Can you work these out from the drawing? Everything is in mm from the part's minimum corner. A direction names the side the tool comes from. Round coordinates to 2 decimals unless told otherwise and drop trailing zeros. Loops run counter-clockwise (first coordinate to the right, second up) from the corner with the lowest first, then second, coordinate; pieces in that order, holes last. Notation, with made-up numbers: M 65.25,-18.5 L 95.25,-18.5 A18 ccw 95.25,9.5 Z; hole C 77.25,12.25 d7. An arc over 180 degrees is marked long. One line per question, with ' | ' between items. Start each with the question number.
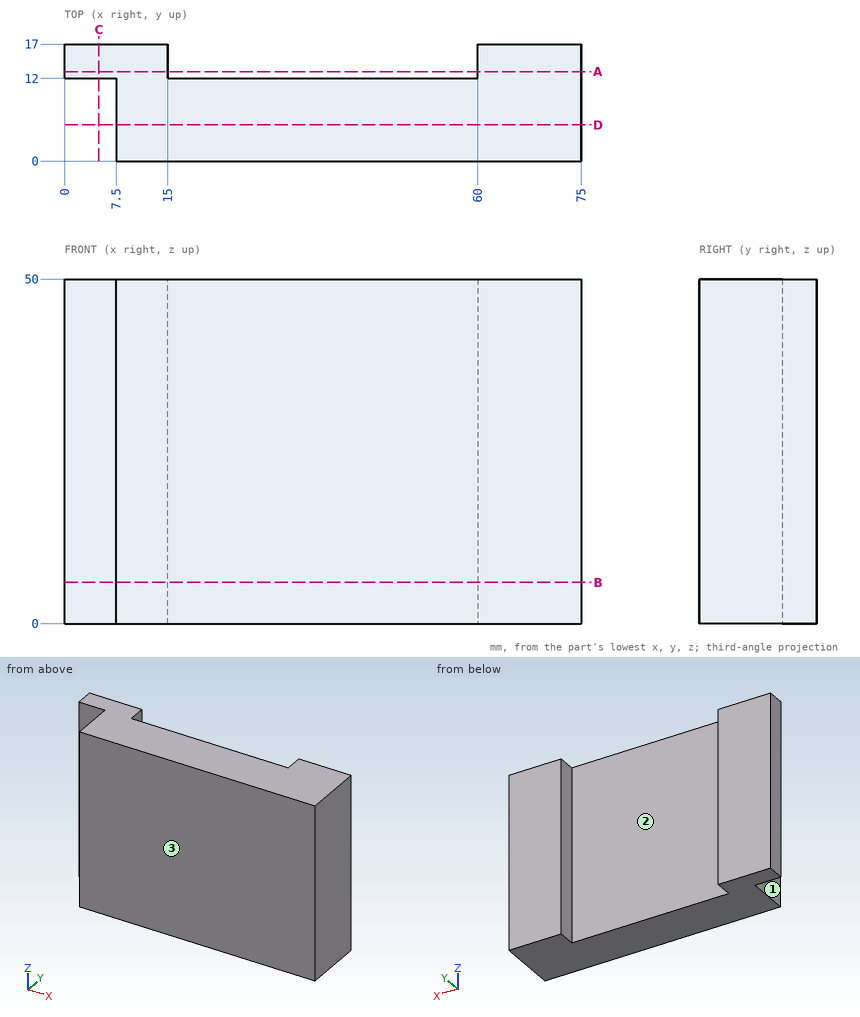
1) Please list where these lines run through material, in increasing order: L1, parallel to X at y = 15, z = 44.5; L2, parallel to X at y = 7, z = 15.5; L3, parallel to Y at x = 22.5, z = 35. Write a range as from..to.
2) I'm going to push flat-ended pins straight in: pin 1 Ø6 at (y, z) = (3.5, 17) entering from -X; pin 2 Ø6 at (x, z) = (3.5, 30) entering from -Y. Where does each tip first touch, or does it pass through?
3) Imagine slicing it at C-C (x = 5). Write out the boundary of the cut face in (y, z).
4) For the marked faces 1, 2 and 3, which set-ups out of +Z, -Z, +X, -X, +Y, -Y let a thin tool reach every point of the face, with its end or its side?
5) Imagine slicing it at D-D (y = 5.25). Write out the boundary of the cut face in (x, z).
6) Imagine slicing it at A-A (y = 13). Write out the boundary of the cut face in (x, z), then the cut area to 3 significant figures.
7) Imagine slicing it at B-B (z = 6). Write out the boundary of the cut face in (x, y), then the cut area to 3 significant figures.
Results are:
1) L1: 0..15, 60..75 | L2: 7.5..75 | L3: 0..12
2) pin 1: x = 7.5 | pin 2: y = 12
3) outline: M 12,0 L 17,0 L 17,50 L 12,50 Z
4) face 1: +Z, -Z, -X, -Y | face 2: +Z, -Z, +Y | face 3: +Z, -Z, +X, -X, -Y
5) outline: M 7.5,0 L 75,0 L 75,50 L 7.5,50 Z
6) outline: M 0,0 L 15,0 L 15,50 L 0,50 Z; M 60,0 L 75,0 L 75,50 L 60,50 Z | area: 1,500 mm²
7) outline: M 0,12 L 7.5,12 L 7.5,0 L 75,0 L 75,17 L 60,17 L 60,12 L 15,12 L 15,17 L 0,17 Z | area: 960 mm²
